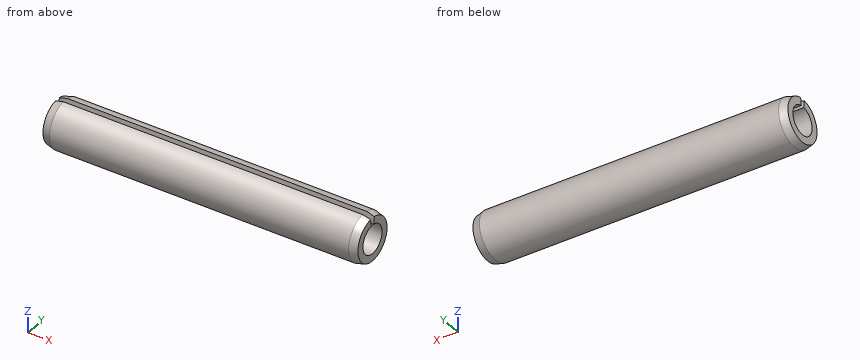
Autodesk Inventor part; units mm, degrees
ref_plane "IDS_WORKPLANE{1}" through (10, 0, 0) normal (1, 0, 0) x (0, 1, 0)
ref_plane "YZ Plane" through (0, 0, 0) normal (1, 0, 0) x (0, 1, 0)
ref_plane "XZ Plane" through (0, 0, 0) normal (0, 1, 0) x (-1, 0, 0)
sketch "Sketch1" plane through (0, 0, 0) normal (0, 0, 1) x (1, 0, 0)
  line L0 (0, 0.9) -> (0, 1.366)
  line L1 (0, 1.366) -> (0.5, 1.5)
  line L2 (0.5, 1.5) -> (19.5, 1.5)
  line L3 (19.5, 1.5) -> (20, 1.366)
  line L4 (20, 1.366) -> (20, 0.9)
  line L5 (20, 0) -> (0, 0)
  line L6 (0, 0.9) -> (20, 0.9)
  line L7 (0, 0.9) -> (0, 0) construction
  line L8 (20, 0.9) -> (20, 0) construction
  line L9 (0, 1.5) -> (0, -0.25)
  line L10 (-2, 0) -> (12, 0)
  dimension "d0" = 20
  dimension "d1" = 3
  dimension "d2" = 1.8
  dimension "d3" = 15
  dimension "d4" = 15
  dimension "d7" = 0.134
  dimension "d8" = 0.134
revolve "Body" add sketch "Sketch1" angle 360 about axis through (20, 0, 0) along (-1, 0, 0)
ref_plane "IDS_WORKPLANE{1}" through (10, 0, 0) normal (1, 0, 0) x (0, 1, 0)
sketch "Sketch2" plane through (10, 0, 0) normal (1, 0, 0) x (0, 1, 0)
  arc A0 (0.188, 1.4882) -> (-0.188, 1.4882) centre (0, 0) ccw
  arc A1 (0.1128, 0.8929) -> (-0.1128, 0.8929) centre (0, 0) ccw
  line L0 (-0.1128, 0.8929) -> (-0.188, 1.4882)
  line L1 (0.1128, 0.8929) -> (0.188, 1.4882)
  line L2 (0, 1.5) -> (0, -0.25)
  line L3 (-0.2193, 0) -> (0.2193, 0)
  dimension "d11" = 1.5
  dimension "d12" = 0.9
  dimension "d14" = 0.6
  dimension "d15" = 7.2
extrude "Cut" cut sketch "Sketch2" against normal mid plane 20
equation "\"d0\" = NLG"
equation "\"d1\" = NND"
equation "\"d2\" = NND - 2 * SD"
equation "\"d3\" = FAWI"
equation "\"d4\" = FAWI"
equation "\"d11\" = 0.5 * NND"
equation "\"d12\" = -SD + 0.5 * NND"
equation "\"d14\" = SD"
equation "\"d5\" = NLG"
equation "\"NND\" = 3"
equation "\"NLG\" = 20"
equation "\"SD\" = 0.6"
equation "\"PHH\" = 0.5"
equation "\"PHH1\" = 0.5"
equation "\"FAWI\" = 15deg"
equation "\"NND1\" = 3.5"
properties part number "ISO 8752 - 3 x 20  A" material "Steel"
Can you work these out from the model? Positions are in its coordinate system, mm. Coordinates: 2 decimals unless noted, no trailing zeros. Write each loop counter-clockwise with the first axis right and the second up, starting at its lowest first coordinate (ties: lowest second). Pieces come first, ordered by that corner, then holes. Notation, with made-up numbers: (10.5, 20.25) - (15.5, 20.25) arc R9 ccw to (15.5, 35.25) - close; hole circle Ø10 at (-11, -20). An arc over 180 degrees is marked (long way). Return JSON: item names as keys, results as strings.
Q1. If we section it at B-B (x = 7): Please give me the cut outline in (y, z), then the cut area to 3 significant figures.
Computed values:
{"outline": "(-0.19, 1.49) arc R1.5 ccw (long way) to (0.19, 1.49) - (0.11, 0.89) arc R0.9 cw (long way) to (-0.11, 0.89) - close", "area": "4.34 mm2"}
Q2. If we section it at A-A (z = 0): Please give me the cut outline in (x, y), then the cut area to 3 significant figures.
Computed values:
{"outline": "(0, -1.37) - (0.5, -1.5) - (19.5, -1.5) - (20, -1.37) - (20, -0.9) - (0, -0.9) - close; (0, 0.9) - (20, 0.9) - (20, 1.37) - (19.5, 1.5) - (0.5, 1.5) - (0, 1.37) - close", "area": "23.9 mm2"}
Q3. Please list where these lines run through material, in increasing order: L1, parallel to Y at x = 11.5, z = 0; L2, parallel to Z at x = 4.75, y = -0.25; L3, parallel to Y at x = 12.25, z = 1. Write a range as from..to.
Computed values:
{"L1": "y = -1.5..-0.9, 0.9..1.5", "L2": "z = -1.48..-0.86, 0.86..1.48", "L3": "y = -1.12..-0.13, 0.13..1.12"}
